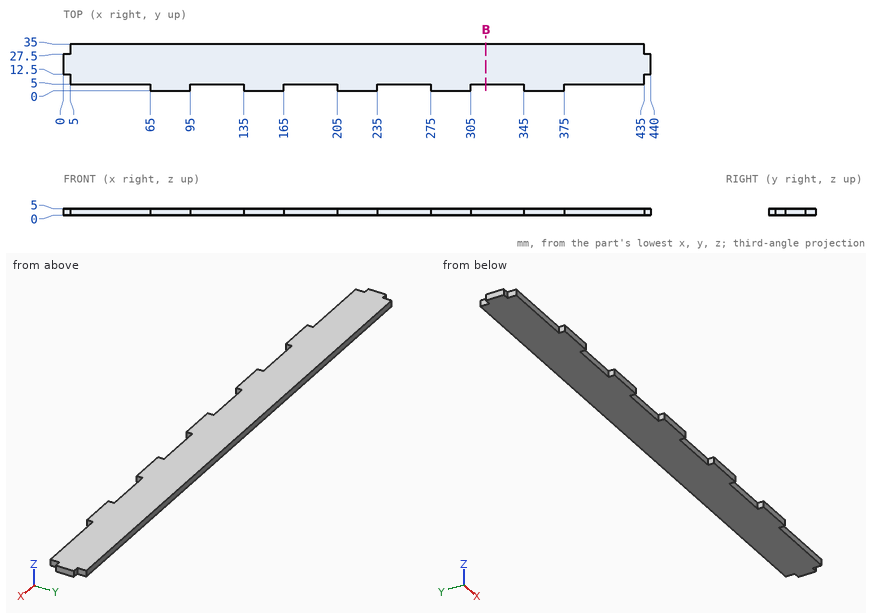
Print and shaded views of the part. All mm, measured from the part's lowest x, y and z. Give positions to 0.01 mm unless a question says otherwise; leave off trailing zeros. Loops run counter-clockwise (first coordinate to the right, second up) from the corner with the lowest first, then second, coordinate; pieces in that order, holes last. Notation, with made-up numbers: (43, 57.25) - (53, 57.25) arc R5 cw to (53, 62.25) - close; hole circle Ø9 at (80.25, 28.25). An arc over 180 degrees is marked (long way). Use a Markdown table: item, result.
(1) Drop flat-ended pins along their axis: pin 1 Ø1.5 at (y, z) = (1.5, 1.5) entering from -X; pin 2 Ø2.5 at (x, z) = (112, 3) entering from -Y; pin 3 Ø1 at (y, z) = (7, 1.5) entering from -X. Give the stop position or say it passes through.
Taken from the geometry:
| item | result |
|---|---|
| pin 1 | x = 65 |
| pin 2 | y = 5 |
| pin 3 | x = 5 |
(2) Wall check: line 1 along X through (y, z) = (3.5, 4.55); line 2 along Y through (x, z) = (171.5, 4.25); line 3 along X through (y, z) = (7.5, 3.65). Give the ranges that are in metal, low to high.
Taken from the geometry:
| item | result |
|---|---|
| line 1 | 65 to 95, 135 to 165, 205 to 235, 275 to 305, 345 to 375 |
| line 2 | 5 to 35 |
| line 3 | 5 to 435 |
(3) Band-saw the part on B-B (x = 316.5). Give the cut face in (y, z), and give its area (3 significant figures).
Taken from the geometry:
| item | result |
|---|---|
| outline | (5, 0) - (35, 0) - (35, 5) - (5, 5) - close |
| area | 150 mm2 |
